Verification items for the finished model (mm, model axes). Give positions to 0.01 mm unless a question says otherwise; leave off trailing zeros. Order: outer loops, then holes, each group sorted by start corner. A loop starts at its lowest first (then second) coordinate and runs counter-clockwise, first axis right, second up.
(1) Sectioned sample at C-C on x = -199.5. Record the cut outline in (y, z) (3 decimals).
(2) Sectioned sample at B-B on z = 1.05. Count the separate pieces of the cut face and the enclosed holes in it, plus the area to 3 significant figures.
(3) Gauge pin test, flat ends, axial feed: pin 1 (1.5 mm diameter, centred on x = -485, z = 1.5, fed in from -Y); pin 2 (1 mm diameter, centred on x = -225.5, z = 1, fed in from -Y) (3 decimals); pin 3 (1.6 mm diameter, centred on x = -378, z = 2, fed in from -Y); pin 4 (4 mm diameter, centred on x = -12.7, y = -21.997, fed in from +Z). Record the tip position at first contact, or that the pin passes through.
(4) Scan lines: L1, parallel to Y at x = -550, z = 1.4 (3 decimals); L2, parallel to X at y = -8, z = 2.3; L3, parallel to Y at x = -321, z = 1.1. Record each from-to range of solid material in increasing order.
(5) Sectioned sample at A-A on x = -469.5. Record the cut outline in (y, z) (1 decimal).
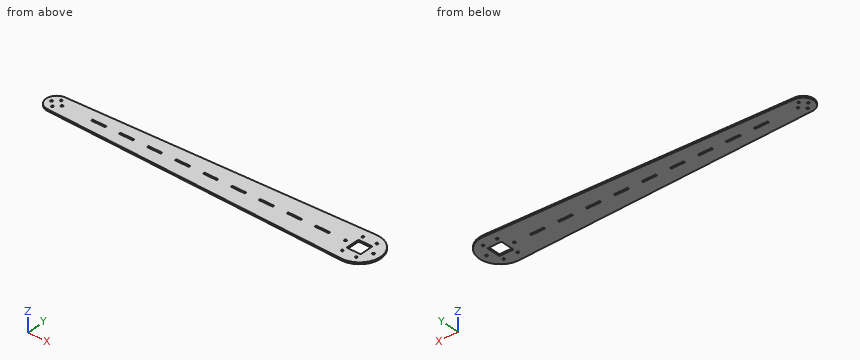
Autodesk Inventor part; units mm, degrees
ref_plane "YZ Plane" through (0, 0, 0) normal (1, 0, 0) x (0, 1, 0)
ref_plane "XZ Plane" through (0, 0, 0) normal (0, 1, 0) x (-1, 0, 0)
ref_plane "XY Plane" through (0, 0, 0) normal (0, 0, 1) x (1, 0, 0)
sketch "Sketch1" plane through (0, 0, 0) normal (0, 0, 1) x (1, 0, 0)
  circle A0 centre (0, 0) radius 31.75
  circle A1 centre (25.4, 0) radius 2.1
  circle A2 centre (-25.4, 0) radius 2.1
  circle A3 centre (12.7, -21.997) radius 2.1
  circle A4 centre (-12.7, -21.997) radius 2.1
  line L0 (12.7, -12.7) -> (12.7, 12.7)
  line L1 (-12.7, -12.7) -> (12.7, -12.7)
  line L2 (-12.7, 12.7) -> (-12.7, -12.7)
  line L3 (12.7, 12.7) -> (-12.7, 12.7)
  circle A5 centre (12.7, 21.997) radius 2.1
  circle A6 centre (-12.7, 21.997) radius 2.1
  circle A7 centre (0, 0) radius 38.1
  line L4 (0, 0) -> (-550, 0)
  circle A8 centre (-550, 0) radius 19.05
  circle A9 centre (-540.475, 0) radius 2
  circle A10 centre (-550, 9.525) radius 2
  circle A11 centre (-559.525, 0) radius 2
  circle A12 centre (-550, -9.525) radius 2
  line L5 (-1.3196, 38.0771) -> (-550.6598, 19.0386)
  line L6 (-1.3196, -38.0771) -> (-550.6598, -19.0386)
  circle A13 centre (12.7, 21.997) radius 2
  circle A14 centre (-12.7, 21.997) radius 2
  circle A15 centre (25.4, 0) radius 2
  circle A16 centre (-25.4, 0) radius 2
  circle A17 centre (12.7, -21.997) radius 2
  circle A18 centre (-12.7, -21.997) radius 2
  line L7 (-486.5, -1.5875) -> (-461.1, -1.5875)
  line L8 (-461.1, -1.5875) -> (-461.1, 1.5875)
  line L9 (-461.1, 1.5875) -> (-486.5, 1.5875)
  line L10 (-486.5, 1.5875) -> (-486.5, -1.5875)
  line L11 (-410.3, -1.5875) -> (-410.3, 1.5875)
  line L12 (-435.7, -1.5875) -> (-410.3, -1.5875)
  line L13 (-410.3, 1.5875) -> (-435.7, 1.5875)
  line L14 (-435.7, 1.5875) -> (-435.7, -1.5875)
  line L15 (-359.5, -1.5875) -> (-359.5, 1.5875)
  line L16 (-384.9, -1.5875) -> (-359.5, -1.5875)
  line L17 (-359.5, 1.5875) -> (-384.9, 1.5875)
  line L18 (-384.9, 1.5875) -> (-384.9, -1.5875)
  line L19 (-308.7, -1.5875) -> (-308.7, 1.5875)
  line L20 (-334.1, -1.5875) -> (-308.7, -1.5875)
  line L21 (-308.7, 1.5875) -> (-334.1, 1.5875)
  line L22 (-334.1, 1.5875) -> (-334.1, -1.5875)
  line L23 (-257.9, -1.5875) -> (-257.9, 1.5875)
  line L24 (-283.3, -1.5875) -> (-257.9, -1.5875)
  line L25 (-257.9, 1.5875) -> (-283.3, 1.5875)
  line L26 (-283.3, 1.5875) -> (-283.3, -1.5875)
  line L27 (-207.1, -1.5875) -> (-207.1, 1.5875)
  line L28 (-232.5, -1.5875) -> (-207.1, -1.5875)
  line L29 (-207.1, 1.5875) -> (-232.5, 1.5875)
  line L30 (-232.5, 1.5875) -> (-232.5, -1.5875)
  line L31 (-156.3, -1.5875) -> (-156.3, 1.5875)
  line L32 (-181.7, -1.5875) -> (-156.3, -1.5875)
  line L33 (-156.3, 1.5875) -> (-181.7, 1.5875)
  line L34 (-181.7, 1.5875) -> (-181.7, -1.5875)
  line L35 (-105.5, -1.5875) -> (-105.5, 1.5875)
  line L36 (-130.9, -1.5875) -> (-105.5, -1.5875)
  line L37 (-105.5, 1.5875) -> (-130.9, 1.5875)
  line L38 (-130.9, 1.5875) -> (-130.9, -1.5875)
  line L39 (-54.7, -1.5875) -> (-54.7, 1.5875)
  line L40 (-80.1, -1.5875) -> (-54.7, -1.5875)
  line L41 (-54.7, 1.5875) -> (-80.1, 1.5875)
  line L42 (-80.1, 1.5875) -> (-80.1, -1.5875)
  point P0 (-486.5, 0)
  point P1 (-473.8, -1.5875)
  point P2 (-423, -1.5875)
  point P3 (-435.7, 0)
  point P4 (-372.2, -1.5875)
  point P5 (-384.9, 0)
  point P6 (-321.4, -1.5875)
  point P7 (-334.1, 0)
  point P8 (-270.6, -1.5875)
  point P9 (-283.3, 0)
  point P10 (-219.8, -1.5875)
  point P11 (-232.5, 0)
  point P12 (-169, -1.5875)
  point P13 (-181.7, 0)
  point P14 (-118.2, -1.5875)
  point P15 (-130.9, 0)
  point P16 (-67.4, -1.5875)
  point P17 (-80.1, 0)
  dimension "d0" = 76.2
  dimension "d1" = 550
  dimension "d2" = 38.1
  dimension "d3" = 4
  dimension "d4" = 9.525
  dimension "d7" = 360
  dimension "d9" = 4
  dimension "d10" = 4
  dimension "d11" = 4
  dimension "d12" = 4
  dimension "d13" = 4
  dimension "d14" = 4
  dimension "d17" = 25.4
  dimension "d18" = 3.175
  dimension "d19" = 76.2
  dimension "d22" = 50.8
extrude "Extrusion1" add sketch "Sketch1" along normal blind 3.175 contours A0 | A7 | A7 L6 A8 L4 L10 L7 L8 L14 L12 L11 L18 L16 L15 L22 L20 L19 L26 L24 L23 L30 L28 L27 L34 L32 L31 L38 L36 L35 L42 L40 L39 | L4 L39 L41 L42 L35 L37 L38 L31 L33 L34 L27 L29 L30 L23 L25 L26 L19 L21 L22 L15 L17 L18 L11 L13 L14 L8 L9 L10 A8 L5 A7 | A8
properties part number "MainArm" material "MDF Medium Density Fiberboard"
Ans:
1. outline: (-31.209, 0) - (31.209, 0) - (31.209, 3.175) - (-31.209, 3.175) - close
2. separate pieces: 1
2. enclosed holes: 20
2. area: 32,800 mm2
3. pin 1: stops at y = -21.34
3. pin 2: stops at y = -30.325
3. pin 3: stops at y = -25.05
3. pin 4: passes through
4. L1: y = -19.061 to -11.525, -7.525 to 7.525, 11.525 to 19.061
4. L2: x = -567.29 to -551.29, -548.71 to -12.7, 12.7 to 37.25
4. L3: y = -27 to -1.59, 1.59 to 27
5. outline: (-21.9, 0) - (-1.6, 0) - (-1.6, 3.2) - (-21.9, 3.2) - close; (1.6, 0) - (21.9, 0) - (21.9, 3.2) - (1.6, 3.2) - close
